```python
from build123d import *
from OCP.BRepAlgoAPI import BRepAlgoAPI_Cut
from OCP.TopTools import TopTools_ListOfShape

# Parameters (mm, degrees)
SALIENTE_EXTRUIR1_DEPTH      = 8
SALIENTE_EXTRUIR1_DEPTH_BACK = 16
CROQUIS1_R                   = 0.8000000000000019
CROQUIS1_R_2                 = 0.8000000000000002
CROQUIS3_W                   = 5.999999999999999
CROQUIS3_H                   = 7.5149398575439825
CORTAR_EXTRUIR1_DEPTH        = 16
CROQUIS4_W                   = 12.500000000000004
CROQUIS4_H                   = 10.000000000000002
CORTAR_EXTRUIR2_DEPTH        = 16
REDONDEO1_R                  = 10
CORTAR_EXTRUIR3_DEPTH        = 39.561831595033986
SALIENTE_EXTRUIR2_START      = -7
SALIENTE_EXTRUIR2_DEPTH      = 7
SALIENTE_EXTRUIR3_START      = -7
SALIENTE_EXTRUIR3_DEPTH      = 7
CORTAR_EXTRUIR4_DEPTH        = 39.561831595033986
SALIENTE_EXTRUIR4_START      = 0.5
SALIENTE_EXTRUIR4_DEPTH      = 0.5
SALIENTE_EXTRUIR5_DEPTH      = 0.5
REDONDEO2_R                  = 1
SALIENTE_EXTRUIR6_DEPTH      = 7.5
SALIENTE_EXTRUIR7_DEPTH      = 7.5
CORTAR_EXTRUIR5_DEPTH        = 6.192871


with BuildPart() as part:
    # Croquis1 → Saliente-Extruir1 (new, two sides: drawn at the far end of the back side and taken through both)
    with BuildSketch(Plane.XY.offset(-SALIENTE_EXTRUIR1_DEPTH_BACK)):
        with BuildLine():
            Line((2.309746663820058, 19.04340690522453), (11.832681853129706, 15.099435825287522))
            ThreePointArc((11.832681853129735, 15.099435825287586), (14.633813116183077, 11.69161014757831), (15.904999780297969, 15.915790146996653))
            Line((15.904999780297969, 15.915790146996654), (16.93335681353175, 18.398814789031395))
            Line((16.93335681353175, 18.398814789031395), (1.029391105834504, 24.985521467228967))
            Line((1.029391105834504, 24.985521467228967), (0, 22.5))
            ThreePointArc((-2.2e-16, 22.5), (-2.078639306967261, 18.611022451034337), (2.3097466638200577, 19.04340690522453))
        make_face()
        with Locations((14.142428516949789, 14.142842730512115)):
            Circle(CROQUIS1_R, mode=Mode.SUBTRACT)
        with Locations((-8e-16, 20)):
            Circle(CROQUIS1_R_2, mode=Mode.SUBTRACT)
    extrude(amount=SALIENTE_EXTRUIR1_DEPTH + SALIENTE_EXTRUIR1_DEPTH_BACK)

    # Croquis3 → Cortar-Extruir1 (cut)
    with BuildSketch(Plane(origin=(8.98354685928157, 21.691268210929703, 0), x_dir=(0.9238986655280315, -0.38263723791016835, 0), z_dir=(0.38263723791016835, 0.9238986655280315, 0))):
        Polygon((-10.15274475820337, -8), (-4.152744758203371, -8), (-4.152744758203371, -0.4850601424560169), (-10.15274475820337, -0.48506014245601775), align=None)
        with Locations((-7.1527447582033705, 12.242530071228009)):
            Rectangle(CROQUIS3_W, CROQUIS3_H)
    extrude(amount=-CORTAR_EXTRUIR1_DEPTH, mode=Mode.SUBTRACT)

    # Croquis4 → Cortar-Extruir2 (cut)
    with BuildSketch(Plane(origin=(8.98354685928157, 21.691268210929703, 0), x_dir=(0.9238986655280315, -0.38263723791016835, 0), z_dir=(0.38263723791016835, 0.9238986655280315, 0))):
        with Locations((8.604634091236255, 4.000000000000001)):
            Rectangle(CROQUIS4_W, CROQUIS4_H)
    extrude(amount=-CORTAR_EXTRUIR2_DEPTH, mode=Mode.SUBTRACT)

    # Redondeo1
    # the kernel refuses this fillet: 10 mm, written as the material it adds along each edge
    with BuildSketch(Plane(origin=(15.90499978029797, 15.915790146996653, 1), x_dir=(0.43937810664982085, -0.898302220523148, 0), z_dir=(0, 0, 1))) as redondeo1_piece_1:
        with BuildLine():
            CenterArc((4.909244259441116, 9.449263834962537), REDONDEO1_R, 228.0261529616087, 22.86990266701423)
            Line((-1.7786689833312208, 2.0147620724265707), (-1.9124272481866686, 1.8660720371758521))
            ThreePointArc((-1.9124272481866686, 1.8660720371758521), (-1.0392674370387214, 0.8750174766821813), (-0.14993294537311094, -0.13236355953110399))
            Line((-0.14993294537311094, -0.13236355953110399), (0.06545659012588191, -0.18898527669924975))
            ThreePointArc((0.06545659012588191, -0.18898527669924975), (0.8182073765735266, -0.06231595874062915), (1.5709581630211649, -0.18898527669925216))
            Line((1.5709581630211649, -0.18898527669925216), (1.636414753147047, 6e-17))
        make_face()
    extrude(amount=7)
    with BuildSketch(Plane(origin=(15.90499978029797, 15.915790146996653, -16), x_dir=(0.43937810664982085, -0.898302220523148, 0), z_dir=(0, 0, 1))) as redondeo1_piece_2:
        with BuildLine():
            CenterArc((4.909244259441116, 9.449263834962537), REDONDEO1_R, 228.0261529616087, 22.86990266701423)
            Line((-1.7786689833312208, 2.0147620724265707), (-1.9124272481866686, 1.8660720371758521))
            ThreePointArc((-1.9124272481866686, 1.8660720371758521), (-1.0392674370387214, 0.8750174766821813), (-0.14993294537311094, -0.13236355953110399))
            Line((-0.14993294537311094, -0.13236355953110399), (0.06545659012588191, -0.18898527669924975))
            ThreePointArc((0.06545659012588191, -0.18898527669924975), (0.8182073765735266, -0.06231595874062915), (1.5709581630211649, -0.18898527669925216))
            Line((1.5709581630211649, -0.18898527669925216), (1.636414753147047, 6e-17))
        make_face()
    extrude(amount=6.999999999999998)
    with BuildSketch(Plane(origin=(-1.1e-16, 22.5, 0.4850601424560175), x_dir=(-0.9451707970750715, -0.3265764295788571, 0), z_dir=(0, 0, -1))) as redondeo1_piece_3:
        with BuildLine():
            CenterArc((4.898646443682852, 9.451707970750716), REDONDEO1_R, 228.06162230808002, 22.877267808488114)
            Line((-1.784663138412825, 2.0130674343443404), (-1.9183293300547388, 1.8642946236162135))
            ThreePointArc((-1.9183293300547388, 1.8642946236162135), (-1.0419879162330352, 0.8738575030467765), (-0.149656347026621, -0.13267621412539496))
            Line((-0.149656347026621, -0.13267621412539496), (0.06531528591577111, -0.18903415941501364))
            ThreePointArc((0.06531528591577111, -0.18903415941501364), (0.8164410739471419, -0.06292699268767933), (1.5675668619785121, -0.1890341594150131))
            Line((1.5675668619785121, -0.1890341594150131), (1.6328821478942839, -5e-17))
        make_face()
    extrude(amount=8.970120284912035)

    # Croquis5 → Cortar-Extruir3 (cut, through all)
    with BuildSketch(Plane.XY.offset(8)):
        with BuildLine():
            Line((2.309746663820078, 19.04340690522458), (2.8048354948987004, 20.238826130100847))
            ThreePointArc((2.8048354948987004, 20.238826130100847), (7.811221113299703, 18.852662916127482), (12.314929423667346, 16.26384911999791))
            Line((12.314929423667346, 16.26384911999791), (11.83268185312971, 15.099435825287534))
            Line((11.83268185312971, 15.099435825287534), (2.309746663820078, 19.04340690522458))
        make_face()
    extrude(amount=-CORTAR_EXTRUIR3_DEPTH, mode=Mode.SUBTRACT)

    # Croquis7 → Saliente-Extruir2 (add)
    with BuildSketch(Plane(origin=(0, 0, -16), x_dir=(-1, 0, 0), z_dir=(0, 0, -1)).offset(SALIENTE_EXTRUIR2_START)):
        with BuildLine():
            Line((-12.314929423667346, 16.26384911999791), (-11.83268185312971, 15.099435825287534))
            Line((-11.83268185312971, 15.099435825287534), (-2.309746663820078, 19.04340690522458))
            Line((-2.309746663820078, 19.04340690522458), (-2.8048354948986987, 20.238826130100847))
            ThreePointArc((-2.8048354948986987, 20.238826130100847), (-7.811221113299688, 18.852662916127446), (-12.314929423667346, 16.26384911999791))
        make_face()
    extrude(amount=SALIENTE_EXTRUIR2_DEPTH)

    # Croquis8 → Saliente-Extruir3 (add)
    with BuildSketch(Plane.XY.offset(8).offset(SALIENTE_EXTRUIR3_START)):
        with BuildLine():
            Line((11.83268185312971, 15.099435825287534), (12.314929423667346, 16.26384911999791))
            ThreePointArc((12.314929423667346, 16.26384911999791), (11.149114957675053, 17.083977118308297), (9.929630744917306, 17.821941587347368))
            ThreePointArc((9.929630744917306, 17.821941587347368), (6.961487524857346, 19.186020427437004), (3.815730334224168, 20.066245940784494))
            ThreePointArc((3.815730334224168, 20.066245940784494), (3.311351692275589, 20.158796440416758), (2.8048354948986964, 20.238826130100843))
            Line((2.8048354948986964, 20.238826130100843), (2.309746663820078, 19.04340690522458))
            Line((2.309746663820078, 19.04340690522458), (11.83268185312971, 15.099435825287534))
        make_face()
    extrude(amount=SALIENTE_EXTRUIR3_DEPTH)

    # Croquis9 → Cortar-Extruir4 (cut, through all)
    with BuildSketch(Plane(origin=(0, 0, -16), x_dir=(-1, 0, 0), z_dir=(0, 0, -1))):
        Polygon((-3.815730334224168, 20.066245940784487), (-3.233645329348107, 18.66076966731441), (-2.309746663820078, 19.04340690522458), (-2.8048354948986987, 20.238826130100847), (-2.8048354948987475, 20.252229554385092), (-3.8209148592802196, 20.078764261810548), align=None)
    extrude(amount=-CORTAR_EXTRUIR4_DEPTH, mode=Mode.SUBTRACT)

    # Croquis10 → Saliente-Extruir4 (add)
    with BuildSketch(Plane.XY.offset(-9.000000000000002).offset(SALIENTE_EXTRUIR4_START)):
        with BuildLine():
            Line((3.233645329348107, 18.66076966731441), (3.8157303342241673, 20.06624594078449))
            ThreePointArc((3.8157303342241673, 20.06624594078449), (6.961487524857336, 19.186020427436976), (9.929630744917306, 17.821941587347368))
            Line((9.929630744917306, 17.821941587347368), (9.24580396443071, 16.170804198329783))
            Line((9.24580396443071, 16.170804198329783), (3.233645329348107, 18.66076966731441))
        make_face()
    extrude(amount=-SALIENTE_EXTRUIR4_DEPTH)

    # Croquis11 → Saliente-Extruir5 (add)
    with BuildSketch(Plane(origin=(0, 0, 1), x_dir=(-1, 0, 0), z_dir=(0, 0, -1))):
        with BuildLine():
            Line((-9.929630744917324, 17.8219415873474), (-9.245803964430717, 16.170804198329783))
            Line((-9.245803964430717, 16.170804198329783), (-3.233645329348109, 18.66076966731441))
            Line((-3.233645329348109, 18.66076966731441), (-3.815730334224181, 20.066245940784526))
            ThreePointArc((-3.815730334224181, 20.066245940784526), (-6.9614875248573655, 19.18602042743705), (-9.929630744917324, 17.8219415873474))
        make_face()
    extrude(amount=SALIENTE_EXTRUIR5_DEPTH)

    # Redondeo2
    redondeo2_edges = [part.edges().sort_by_distance(p)[0] for p in [
        (10.202397059206133, 18.48055086214986, -9.000000000000002),
        (10.202397059206136, 18.48055086214986, 1),
    ]]
    fillet(redondeo2_edges, radius=REDONDEO2_R)

    # Croquis12 → Saliente-Extruir6 (add)
    with BuildSketch(Plane.XY.offset(8)):
        Polygon((11.83268185312971, 15.099435825287534), (11.436504054366878, 14.142842730512099), (11.37624481953794, 13.997343492256391), (2.7772082957563384, 17.558677334283267), (3.233645329348107, 18.66076966731441), align=None)
    extrude(amount=-SALIENTE_EXTRUIR6_DEPTH)

    # Croquis13 → Saliente-Extruir7 (add)
    with BuildSketch(Plane(origin=(0, 0, -16), x_dir=(-1, 0, 0), z_dir=(0, 0, -1))):
        Polygon((-3.233645329348117, 18.660769667314405), (-2.7772082957563384, 17.558677334283267), (-11.37624481953794, 13.997343492256391), (-11.83268185312971, 15.099435825287534), align=None)
    extrude(amount=-SALIENTE_EXTRUIR7_DEPTH)


with BuildPart() as cortar_extruir5_tool:
    # Croquis15 → Cortar-Extruir5 (new body)
    with BuildSketch(Plane(origin=(8.98354685928157, 21.691268210929703, 0), x_dir=(0.9238986655280315, -0.38263723791016835, 0), z_dir=(0.38263723791016835, 0.9238986655280315, 0))):
        with BuildLine():
            Line((8.604634091236257, 9.000000000000002), (8.604634091236257, -1))
            Line((8.604634091236257, -1), (3.3546340912362544, -1))
            ThreePointArc((3.3546340912362544, -1), (2.6475273100497065, -0.7071067811865478), (2.354634091236254, 1.2e-16))
            Line((2.354634091236254, 1.2e-16), (2.354634091236254, 8))
            ThreePointArc((2.354634091236254, 8), (2.6475273100497057, 8.70710678118655), (3.3546340912362544, 9.000000000000002))
            Line((3.3546340912362544, 9.000000000000002), (8.604634091236257, 9.000000000000002))
        make_face()
    extrude(amount=-CORTAR_EXTRUIR5_DEPTH)


with BuildPart() as part_1:
    add(part.part)

    # Cortar-Extruir5: cut by cortar_extruir5_tool, with a tolerance
    cortar_extruir5_stock = TopTools_ListOfShape()
    cortar_extruir5_stock.Append(part_1.part.wrapped)
    cortar_extruir5_tools = TopTools_ListOfShape()
    cortar_extruir5_tools.Append(cortar_extruir5_tool.part.wrapped)
    cortar_extruir5_cut = BRepAlgoAPI_Cut()
    cortar_extruir5_cut.SetArguments(cortar_extruir5_stock)
    cortar_extruir5_cut.SetTools(cortar_extruir5_tools)
    cortar_extruir5_cut.SetFuzzyValue(0.00001)
    cortar_extruir5_cut.Build()
    add(Compound.cast(cortar_extruir5_cut.Shape()).solids(), mode=Mode.REPLACE)


solid = part_1.part
```
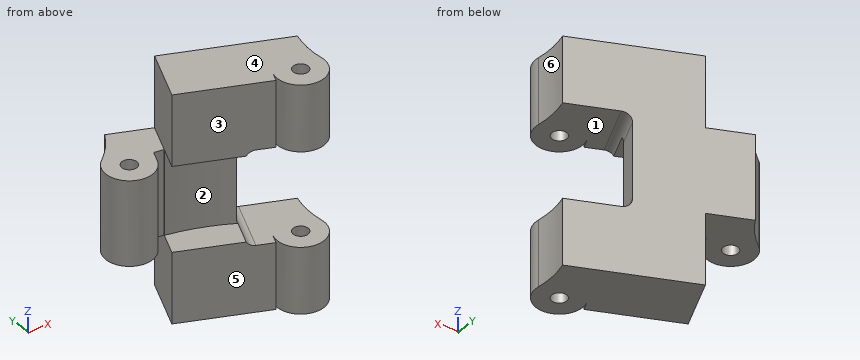
Here's how the part is built. I have some questions about the finished solid (model axes, mm). Face numbers are marked on the shaded views. A direction names the side the tool comes from. Give positions to 0.01 mm unless a question says otherwise; leave off trailing zeros. Order: outer loops, then holes, each group sorted by start corner. A loop starts at its lowest first (then second) coordinate and runs counter-clockwise, first axis right, second up. Notation, with made-up numbers: M -35.75,71.5 L 4.25,71.5 A31 ccw 4.25,108.5 Z; hole C 11.25,67 d7. An arc over 180 degrees is marked long. Use a Markdown table: item, result. Add a question column.
1. On a 3-axis mill with a long thin cutter (end or side, diameter ignored), from which of +Z, -Z, +X, -X, +Y, -Y can I reach the whole of each face in a straight line? I mean the marked faces 1, 2 and 3. Say none if no direction works.
2. If we mould it in two halves opening along Y, with no side actions, what happens to the marked faces 4, 5 and 6? For each: +Y half, -Y half, draft (parallel to the pull), parting line (faces both ways), or undercut.
3. I need wall thicknesses on probe 1 along Z at (x, y) = (1, 20.75); probe 2 along Y at (x, z) = (0, -2.25); probe 3 along Y at (x, z) = (15, 4.25). Which ranges of each line are inside material? Lowest first, please. Write a range as from..to.
4. Suppose I cut it at D-D (x = 0). List the corners of the cut face in (y, z) for me, and give its area (3 significant figures).
5. For pin 1 Ø5 at (x, z) = (6, -3) entering from -Y; pin 2 Ø6 at (x, z) = (12, 4.5) entering from +Y; pin 3 Ø4 at (x, y) = (1, 21) entering from +Z, each with a flat end and sliding along its axis, tell me the tip position at first contact or that it passes through.
6. Suppose I cut it at B-B (x = 3.25). List the corners of the cut face in (y, z) for me, and give its area (3 significant figures).
7. Suppose I cut it at C-C (x = 13). List the corners of the cut face in (y, z) for me.
Results list:
| question | item | result |
|---|---|---|
| 1 | face 1 | +X, -Y |
| 1 | face 2 | -Y |
| 1 | face 3 | +Z, -Z, -X, -Y |
| 2 | face 4 | draft |
| 2 | face 5 | -Y half |
| 2 | face 6 | undercut |
| 3 | probe 1 | z = -8.49..0.49 |
| 3 | probe 2 | y = 17.5..19.2, 20.8..23.47 |
| 3 | probe 3 | y = 11.79..19.2 |
| 4 | outline | M 17.5,-8.49 L 19.2,-8.49 L 19.2,0.49 L 17.5,0.49 Z; M 20.8,-8.49 L 23.47,-8.49 L 23.47,0.49 L 20.8,0.49 Z |
| 4 | area | 39.2 mm² |
| 5 | pin 1 | stops at y = 18.55 |
| 5 | pin 2 | stops at y = 21.68 |
| 5 | pin 3 | stops at z = 0.49 |
| 6 | outline | M 17.36,-16 L 18.7,-16 L 18.7,-8.5 L 17.36,-8.5 Z; M 17.36,0.5 L 18.7,0.5 L 18.7,8 L 17.36,8 Z; M 20.18,-8.49 L 24.07,-8.49 L 24.07,0.49 L 20.18,0.49 Z |
| 6 | area | 55.0 mm² |
| 7 | outline | M 11.92,-16 L 20.03,-16 L 20.03,-9 L 11.92,-9 Z; M 11.92,1 L 20.03,1 L 20.03,8 L 11.92,8 Z |
